```python
from build123d import *

# Parameters (mm, degrees)
F0_R     = 5.55625
F0_R_2   = 2.794
F1_DEPTH = 260.35
F3_R     = 2.778125
F4_DEPTH = 2.286
F5_R     = 1.5875
F6_DEPTH = 2.286


with BuildPart() as f1:
    # F0 (on Front) → F1 (new body)
    with BuildSketch(Plane.XZ):
        Circle(F0_R)
        Circle(F0_R_2, mode=Mode.SUBTRACT)
    extrude(amount=F1_DEPTH)

    # F3 (on offset) → F4 (cut)
    with BuildSketch(Plane.XY.offset(6.35)):
        with Locations((0, -6.35)):
            Circle(F3_R)
    extrude(amount=-F4_DEPTH, mode=Mode.SUBTRACT)

    # F5 (on face) → F6 (cut)
    with BuildSketch(Plane.XY.offset(4.064)):
        with Locations((0, -6.35)):
            Circle(F5_R)
    extrude(amount=-F6_DEPTH, mode=Mode.SUBTRACT)

    # F7 (on Top) → F8 (revolve, cut)
    with BuildSketch(Plane.XY):
        Polygon((6.375642, -259.197921), (3.892762, -260.484248), (6.375642, -261.022687), align=None)
    revolve(axis=Axis((0, -258.301109, 0), (0, 1, 0)), mode=Mode.SUBTRACT)


solid = f1.part
```
Check sheet for the modelled part. Datum: model origin and axes. Units: mm. A direction names the side the tool comes from. Coordinates: 2 decimals unless noted, no trailing zeros. Loops run counter-clockwise (first coordinate to the right, second up) from the corner with the lowest first, then second, coordinate; pieces in that order, holes last.
1) Sectioned sample at A-A (z = 0). Record the boundary of the cut face in (x, y).
2) Sectioned sample at B-B (y = -68). Record the boundary of the cut face in (x, z).
3) Access from +Z, -Z, +X, -X, +Y, -Y to the whole of each face (thin tool, end or side, straight path). Record for faces 4 (the face through (5.3, -127.99, 1.67)), 5 (the face through (1.494, -4.007, 4.657)).
4) Release check for a two-part mould opening along Z. For faces 1 (the face through (1, -8, 4.064)), 2 (the face through (-3, 0, -1)), 3 (the face through (-2.217, -128.353, -1.7)) record: released by +Z, released by -Z, zero draft, split by the parting line, or undercut.
5) Gauge pin test, flat ends, axial feed: pin 1 (3 mm diameter, centred on x = -2, y = -119, fed in from -Z); pin 2 (1.7 mm diameter, centred on x = 1, y = -6, fed in from +Z); pin 3 (4 mm diameter, centred on x = 3, y = -120.5, fed in from +Z). Record the tip position at first contact, or that the pin passes through.
6) Material ranges on probe 1 along X at (y, z) = (-15, -0.25); probe 2 along Z at (x, y) = (0, -202); probe 3 along Z at (x, y) = (-0.5, -168), recorded low to high.
Check sheet entries:
1. outline: (-5.56, -259.62) - (-4.15, -260.35) - (-2.79, -260.35) - (-2.79, 0) - (-5.56, 0) - close; (2.79, -260.35) - (4.15, -260.35) - (5.56, -259.62) - (5.56, 0) - (2.79, 0) - close
2. outline: circle Ø11.11 at (0, 0); hole circle Ø5.59 at (0, 0)
3. face 4: +Y, -Y
3. face 5: +Z
4. face 1: released by +Z
4. face 2: zero draft
4. face 3: undercut
5. pin 1: stops at z = -5.53
5. pin 2: stops at z = 4.06
5. pin 3: stops at z = 5.47
6. probe 1: x = -5.55 to -2.78, 2.78 to 5.55
6. probe 2: z = -5.56 to -2.79, 2.79 to 5.56
6. probe 3: z = -5.53 to -2.75, 2.75 to 5.53
